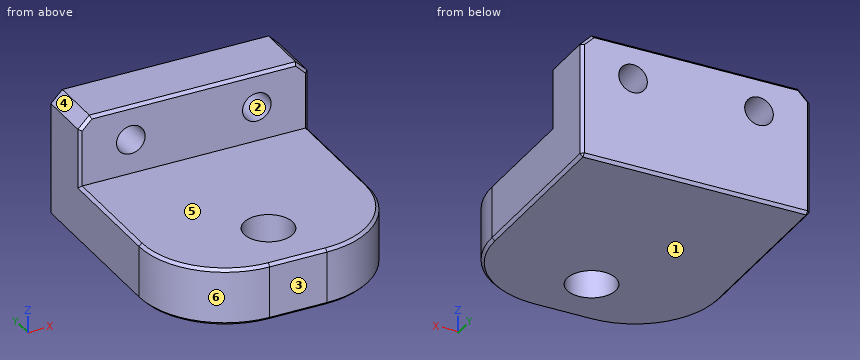
```python
from build123d import *

# Parameters (mm, degrees)
SKETCH_1_W          = 40
SKETCH_1_H          = 45
EXTRUDE_1_DEPTH     = 5
SKETCH_2_W          = 40
SKETCH_2_H          = 10
EXTRUDE_2_DEPTH     = 12
HOLE_WIZARD_M10_1_D = 8.5
HOLE_WIZARD_M6_1_D  = 5
FILLET_1_R          = 15
CHAMFER_1_SIZE      = 2
CHAMFER_2_SIZE      = 0.5


with BuildPart() as part:
    # 草图1 → 凸台-拉伸1 (new, symmetric)
    with BuildSketch(Plane.XY):
        Rectangle(SKETCH_1_W, SKETCH_1_H)
    extrude(amount=EXTRUDE_1_DEPTH, both=True)

    # 草图2 → 凸台-拉伸2 (add)
    with BuildSketch(Plane.XY.offset(5)):
        with Locations((0, 17.5)):
            Rectangle(SKETCH_2_W, SKETCH_2_H)
    extrude(amount=EXTRUDE_2_DEPTH)

    # M10 螺纹孔1 (through all)
    with Locations(Plane(origin=(0, 0, -5), x_dir=(-1, 0, 0), z_dir=(0, 0, -1))):
        with Locations((0, -12.5)):
            Hole(HOLE_WIZARD_M10_1_D / 2)

    # M6 螺纹孔1 (through all)
    with Locations(Plane(origin=(0, 12.5, 0), x_dir=(-1, 0, 0), z_dir=(0, -1, 0))):
        with Locations((-11, -11), (11, -11)):
            Hole(HOLE_WIZARD_M6_1_D / 2)

    # 圆角1
    fillet_1_edges = [part.edges().sort_by_distance(p)[0] for p in [
        (20, -22.5, 0),
        (-20, -22.5, 0),
    ]]
    fillet(fillet_1_edges, radius=FILLET_1_R)

    # 倒角1
    chamfer_1_edges = [part.edges().sort_by_distance(p)[0] for p in [
        (-20, 17.5, 17),
        (20, 17.5, 17),
    ]]
    chamfer(chamfer_1_edges, length=CHAMFER_1_SIZE)

    # 倒角2
    chamfer_2_edges = [part.edges().sort_by_distance(p)[0] for p in [
        (-20, 2.5, 5),
        (0, -22.5, -5),
        (0, -22.5, 5),
        (20, 7.5, -5),
        (15.606601718, -18.106601718, -5),
        (-15.606601718, -18.106601718, -5),
        (20, 2.5, 5),
        (15.606601718, -18.106601718, 5),
        (-15.606601718, -18.106601718, 5),
        (-20, 7.5, -5),
        (0, 22.5, -5),
        (0, 12.5, 17),
        (0, 22.5, 17),
        (20, 12.5, 10),
        (-20, 12.5, 10),
        (19, 12.5, 16),
        (-19, 12.5, 16),
        (-20, 22.5, 5),
        (20, 22.5, 5),
        (19, 22.5, 16),
        (-19, 22.5, 16),
    ]]
    chamfer(chamfer_2_edges, length=CHAMFER_2_SIZE)


solid = part.part
```
Read the model definition and answer for the solid it produces. Units are mm, in the model's axes. Face numbers are marked on the shaded views. A direction names the side the tool comes from. Give positions to 0.01 mm unless a question says otherwise; leave off trailing zeros. Order: outer loops, then holes, each group sorted by start corner. A loop starts at its lowest first (then second) coordinate and runs counter-clockwise, first axis right, second up. Notation, with made-up numbers: (-1.75, 83) -> (34.25, 83) arc R29 ccw to (34.25, 122) -> close; hole circle Ø3 at (5, 50.25). An arc over 180 degrees is marked (long way). Write item = value, one per line.
1. Given pin 1 (4.5 mm diameter, centred on x = -11, z = 11, fed in from +Y); pin 2 (6 mm diameter, centred on x = -2, z = 11, fed in from -Y); pin 3 (8 mm diameter, centred on x = -7, y = -6, fed in from +Z); pin 4 (10 mm diameter, centred on x = 14, z = 8, fed in from -Y), each flat-ended and moving along its own axis, determine where each tip first touches the part or whether it passes through.
Numbers:
pin_1 = through
pin_2 = 12.5
pin_3 = 5
pin_4 = -21.48
2. A cutting plane is placed at B-B, the plane z = 11. Write down the section's boundary in (x, y).
Numbers:
outline = (-20, 13) -> (-19.5, 12.5) -> (-13.5, 12.5) -> (-13.5, 22.5) -> (-19.5, 22.5) -> (-20, 22) -> close; (-8.5, 12.5) -> (8.5, 12.5) -> (8.5, 22.5) -> (-8.5, 22.5) -> close; (13.5, 12.5) -> (19.5, 12.5) -> (20, 13) -> (20, 22) -> (19.5, 22.5) -> (13.5, 22.5) -> close
3. The mould has two halves that part along Z. Classify the marked faces 1, 2, 3 and 4: +Z half, -Z half, draft (parallel to the pull), parting line (faces both ways), or undercut.
Numbers:
face_1 = -Z half
face_2 = undercut
face_3 = draft
face_4 = +Z half
4. A cutting plane is placed at D-D, the plane z = 3.5. Write down the section's boundary in (x, y), and give its area (3 significant figures).
Numbers:
outline = (-20, -7.5) arc R15 ccw to (-5, -22.5) -> (5, -22.5) arc R15 ccw to (20, -7.5) -> (20, 22) -> (19.5, 22.5) -> (-19.5, 22.5) -> (-20, 22) -> close; hole circle Ø8.5 at (0, -12.5)
area = 1,650 mm²
5. A cutting plane is placed at A-A, the plane x = 0. Write down the section's boundary in (y, z).
Numbers:
outline = (-22.5, -4.5) -> (-22, -5) -> (-16.75, -5) -> (-16.75, 5) -> (-22, 5) -> (-22.5, 4.5) -> close; (-8.25, -5) -> (22, -5) -> (22.5, -4.5) -> (22.5, 16.5) -> (22, 17) -> (13, 17) -> (12.5, 16.5) -> (12.5, 5) -> (-8.25, 5) -> close
6. For the marked faces 5 and 6, determine the directions among +Z, -Z, +X, -X, +Y, -Y from which every point of the face is accessible in a straight line to the end or side of a thin tool.
Numbers:
face_5 = +Z, +X, -X, -Y
face_6 = +Z, -Z, -X, -Y
7. A cutting plane is placed at C-C, the plane y = 19. Write down the section's boundary in (x, z).
Numbers:
outline = (-20, -4.5) -> (-19.5, -5) -> (19.5, -5) -> (20, -4.5) -> (20, 15) -> (18, 17) -> (-18, 17) -> (-20, 15) -> close; hole circle Ø5 at (-11, 11); hole circle Ø5 at (11, 11)
8. Straight lines are drawn through the part: line 1 along X through (y, z) = (20, 11); line 2 along Z through (x, y) = (11, 15); line 3 along X through (y, z) = (21, 10.5). For each, find the intervals that lie inside material, in ascending order.
Numbers:
line_1 = -20 to -13.5, -8.5 to 8.5, 13.5 to 20
line_2 = -5 to 8.5, 13.5 to 17
line_3 = -20 to -13.45, -8.55 to 8.55, 13.45 to 20
